from build123d import *

# Parameters (mm, degrees)
SKETCH1_R           = 25.4
SKETCH1_R_2         = 20.066
BOSS_EXTRUDE1_DEPTH = 50.8
BOSS_EXTRUDE2_DEPTH = 31.75
SKETCH3_W           = 25.4
SKETCH3_H           = 25.4
CUT_EXTRUDE1_DEPTH  = 38.1
SKETCH4_R           = 2.50825
CUT_EXTRUDE2_DEPTH  = 31.75
LPATTERN1_COUNT     = 3
LPATTERN1_PITCH     = 12.7


with BuildPart() as part:
    # Sketch1 → Boss-Extrude1 (new body)
    with BuildSketch(Plane.XY):
        Circle(SKETCH1_R)
        Circle(SKETCH1_R_2, mode=Mode.SUBTRACT)
    extrude(amount=BOSS_EXTRUDE1_DEPTH)

    # Sketch2 → Boss-Extrude2 (add)
    with BuildSketch(Plane.XY.offset(50.8)):
        with BuildLine():
            Line((-19.827868645, 15.875), (-63.5, 15.875))
            Line((-63.5, 15.875), (-63.5, -15.875))
            Line((-63.5, -15.875), (-19.827868645, -15.875))
            ThreePointArc((-19.827868645, -15.875), (-25.4, 0), (-19.827868645, 15.875))
        make_face()
    extrude(amount=-BOSS_EXTRUDE2_DEPTH)

    # Sketch3 → Cut-Extrude1 (cut)
    with BuildSketch(Plane.ZY.offset(63.5)):
        with Locations((34.925, 0)):
            Rectangle(SKETCH3_W, SKETCH3_H)
    extrude(amount=-CUT_EXTRUDE1_DEPTH, mode=Mode.SUBTRACT)

    # Sketch4 → Cut-Extrude2 (cut)
    with BuildSketch(Plane.XY.offset(50.8)):
        with Locations((-57.15, 6.35)):
            Circle(SKETCH4_R)
        with Locations((-57.15, -6.35)):
            Circle(SKETCH4_R)
    cut_extrude2 = extrude(amount=-CUT_EXTRUDE2_DEPTH, mode=Mode.SUBTRACT)

    # LPattern1: Cut-Extrude2 ×3
    with Locations(*[(i * LPATTERN1_PITCH, 0, 0) for i in range(1, LPATTERN1_COUNT)]):
        add(cut_extrude2, mode=Mode.SUBTRACT)


solid = part.part
Work out the finished part from the listing and answer in its coordinate system (mm). A direction names the side the tool comes from. Round coordinates to 2 decimals unless told otherwise and drop trailing zeros. Loops run counter-clockwise (first coordinate to the right, second up) from the corner with the lowest first, then second, coordinate; pieces in that order, holes last. Notation, with made-up numbers: M -12,86.5 L -8,86.5 A24 cw -8,125.5 Z; hole C 33,57 d9. An arc over 180 degrees is marked long. One line per question, with ' | ' between items. Start each with the question number.
(1) A cutting plane is placed at C-C on x = 0. Write down the section's boundary in (y, z), plus the area to 3 significant figures.
(2) Find the intervals of material crossed by line 1 (Y direction, x = -57.15, z = 21.15) (3 decimals); line 2 (Z direction, x = -55, y = 1) (3 decimals); line 3 (X direction, y = -6, z = 49), in increasing order.
(3) A cutting plane is placed at A-A on y = 0. Write down the section's boundary in (x, z) (3 decimals).
(4) Flat-ended cylindrical pins translate along their axes: pin 1 Ø2 at (x, z) = (5.5, 32.5) entering from -Y; pin 2 Ø5 at (x, z) = (-18.5, 36.5) entering from -Y; pin 3 Ø20.5 at (x, z) = (-47.5, 30) entering from -Y (3 decimals); pin 4 Ø6 at (x, y) = (-31.75, 6.35) entering from +Z. Find the tip coordinate at first contact, or state that the pin passes through.
(5) A cutting plane is placed at D-D on x = -57.15. Write down the section's boundary in (y, z) (3 decimals).
(6) A cutting plane is placed at B-B on x = -36. Write down the section's boundary in (y, z) (3 decimals), plus the area to 3 significant figures.
(7) A tool of negligible diameter and unlimited length cuts with its end or side. For faces 1 (the face through (-41, 15.875, 35)), 2 (the face through (-45, 0, 22.225)), 3 (the face through (-42, -15.875, 35)), from which of +Z, -Z, +X, -X, +Y, -Y can it reach the whole face along a straight path? Write none if from no direction.
(8) For a pull along Z with two mould halves and no side action, classify faces 4 (the face through (-4.3, -19.6, 25)), 5 (the face through (19, 8, 0)), 6 (the face through (-45, -12.7, 35)) as released by +Z, released by -Z, zero draft, split by the parting line, or undercut.
Geometry check:
1) outline: M -25.4,0 L -20.07,0 L -20.07,50.8 L -25.4,50.8 Z; M 20.07,0 L 25.4,0 L 25.4,50.8 L 20.07,50.8 Z | area: 542 mm²
2) line 1: y = -15.875 to -8.858, -3.842 to 3.842, 8.858 to 15.875 | line 2: z = 19.05 to 22.225, 47.625 to 50.8 | line 3: x = -63.5 to -59.63, -54.67 to -46.93, -41.97 to -34.23, -29.27 to -19.15, 19.15 to 24.68
3) outline: M -63.5,19.05 L -25.4,19.05 L -25.4,0 L -20.066,0 L -20.066,50.8 L -63.5,50.8 L -63.5,47.625 L -25.4,47.625 L -25.4,22.225 L -63.5,22.225 Z; M 20.066,0 L 25.4,0 L 25.4,50.8 L 20.066,50.8 Z
4) pin 1: stops at y = -25 | pin 2: stops at y = -19.73 | pin 3: stops at y = -15.875 | pin 4: stops at z = 50.8
5) outline: M -15.875,19.05 L -8.858,19.05 L -8.858,22.225 L -12.7,22.225 L -12.7,47.625 L -8.858,47.625 L -8.858,50.8 L -15.875,50.8 Z; M -3.842,19.05 L 3.842,19.05 L 3.842,22.225 L -3.842,22.225 Z; M -3.842,47.625 L 3.842,47.625 L 3.842,50.8 L -3.842,50.8 Z; M 8.858,19.05 L 15.875,19.05 L 15.875,50.8 L 8.858,50.8 L 8.858,47.625 L 12.7,47.625 L 12.7,22.225 L 8.858,22.225 Z
6) outline: M -15.875,19.05 L 15.875,19.05 L 15.875,50.8 L -15.875,50.8 Z; hole M -12.7,22.225 L 12.7,22.225 L 12.7,47.625 L -12.7,47.625 Z | area: 363 mm²
7) face 1: +Z, -Z, -X, +Y | face 2: -X | face 3: +Z, -Z, -X, -Y
8) face 4: zero draft | face 5: released by -Z | face 6: undercut
